Read the model definition and answer for the solid it produces. Units are mm, in the model's axes. A direction names the side the tool comes from. Coordinates: 2 decimals unless noted, no trailing zeros. Loops run counter-clockwise (first coordinate to the right, second up) from the corner with the lowest first, then second, coordinate; pieces in that order, holes last. Notation, with made-up numbers: (18, 41.5) -> (28, 41.5) arc R32 ccw to (28, 80.5) -> close; hole circle Ø10 at (-17, -15). An arc over 180 degrees is marked (long way). Answer as a JSON object with one key per item and string values. Group by question number.
Q1. The part is cut by section C-C on z = -3.5. Write down the section's boundary in (x, y).
Q2. The part is cut by section D-D on z = 2. Write down the section's boundary in (x, y).
Q3. For faces 5 (the flat face through (-20, 2, -2)), 6 (the flat face through (-27, 2, -5)), 7 (the cylindrical face through (29.43, 5.01, -9.4)), 8 (the flat face through (7, 2, 0)), determine the directions among +Z, -Z, +X, -X, +Y, -Y from which every point of the face is accessible in a straight line to the end or side of a thin tool.
Q4. Each of these flat-tipped pins is pushed along its axis until it touches: P1, Ø1.2, axis at x = 8.5, y = 2, coming from the +Z side; P2, Ø3, axis at y = 1, z = -1.5, coming from the +X side; P3, Ø2, axis at y = 2, z = -3.5, coming from the -X side; P4, Ø1.5, axis at y = 2, z = 2.5, coming from the +X side. Where does it stop, or does it pass through?
Q5. The part is cut by section B-B on x = 13. Write down the section's boundary in (y, z).
Q6. Determine the mould class of faces 1 (the flat face through (15, 2, -2)), 2 (the flat face through (-11, 4, -3)), 3 (the flat face through (0, 2, -3)), 4 (the flat face through (8, 0, -2)) for opening direction X: released by +X, released by -X, zero draft, split by the parting line, or undercut.
Q7. The part is cut by section A-A on y = 1.85. Write down the section's boundary in (x, z), and give its area (3 significant figures).
Q8. Straight lines are drawn through the part: line 1 along X through (y, z) = (0.4, -4.75); line 2 along Y through (x, z) = (17, -8.5); line 3 along Z through (x, y) = (-22, 1.1). For each, find the intervals that lie inside material, in ascending order. Write a range as [from, to].
Autodesk Inventor part; units mm, degrees
ref_plane "YZ Plane" through (0, 0, 0) normal (1, 0, 0) x (0, 1, 0)
ref_plane "XZ Plane" through (0, 0, 0) normal (0, 1, 0) x (-1, 0, 0)
ref_plane "XY Plane" through (0, 0, 0) normal (0, 0, 1) x (1, 0, 0)
sketch "Эскиз1" plane through (0, 0, 0) normal (0, 1, 0) x (-1, 0, 0)
  line L0 (0, 0) -> (-15, 0)
  line L1 (-15, 0) -> (-15, -5)
  line L2 (-15, -5) -> (0, -5)
  line L3 (0, -5) -> (0, 0)
  dimension "d0" = 5
  dimension "d1" = 15
extrude "Выдавливание1" add sketch "Эскиз1" along normal blind 4
sketch "Эскиз2" plane through (0, 4, 0) normal (0, 1, 0) x (1, 0, 0)
  line L0 (-10, -5) -> (30, -5)
  line L1 (30, -5) -> (30, 10)
  line L2 (30, 10) -> (-10, 10)
  line L3 (-10, 10) -> (-10, -5)
  line L4 (-10, 2.5) -> (-4.0843, 2.5)
  line L5 (0, 5) -> (0, 0)
  line L6 (0, 2.5) -> (15, 2.5)
  line L7 (15, 0) -> (15, 5)
  dimension "d4" = 10
  dimension "d5" = 5
  dimension "d6" = 15
extrude "Выдавливание2" add sketch "Эскиз2" along normal blind 2
fillet "Сопряжение1" radius 2 2 edges at (30, 5, 5) (30, 5, -10)
mirror "Зеркальное отражение1" about plane through (-10, 4, -10) normal (-1, 0, 0)
properties part number "верхняя защелка башни"
Final values:
{
 "1": {"outline": "(-50, 4) -> (-35, 4) -> (-35, 0) -> (-20, 0) -> (-20, 4) -> (0, 4) -> (0, 0) -> (15, 0) -> (15, 4) -> (30, 4) -> (30, 6) -> (-50, 6) -> close"},
 "2": {"outline": "(-50, 4) -> (30, 4) -> (30, 6) -> (-50, 6) -> close"},
 "3": {"face 5": "+Z, -Z, -Y", "face 6": "-Z, +X, -X, -Y", "face 7": "-Z, +X, +Y, -Y", "face 8": "+Z, +X, -X, -Y"},
 "4": {"P1": "stops at z = 0", "P2": "stops at x = 15", "P3": "stops at x = -35", "P4": "passes through"},
 "5": {"outline": "(0, -5) -> (4, -5) -> (4, -10) -> (6, -10) -> (6, 5) -> (4, 5) -> (4, 0) -> (0, 0) -> close"},
 "6": {"face 1": "released by +X", "face 2": "undercut", "face 3": "undercut", "face 4": "zero draft"},
 "7": {"outline": "(-35, -5) -> (-20, -5) -> (-20, 0) -> (-35, 0) -> close; (0, -5) -> (15, -5) -> (15, 0) -> (0, 0) -> close", "area": "150 mm2"},
 "8": {"line 1": "x = [-35, -20], [0, 15]", "line 2": "y = [4, 6]", "line 3": "z = [-5, 0]"}
}
